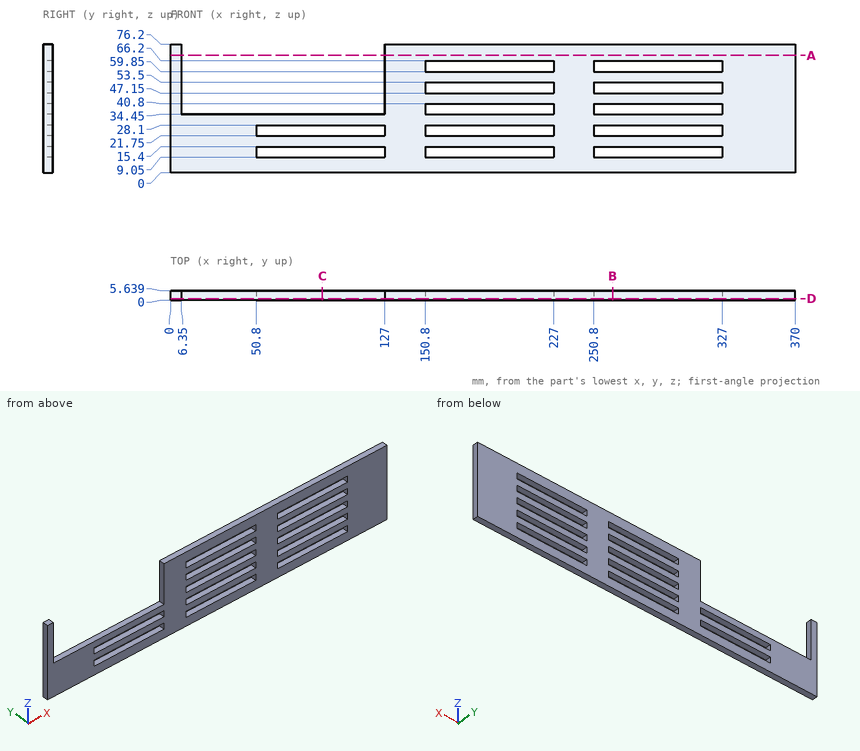
Part print with two shaded views. Sizes in mm from the minimum x, y, z corner. Round coordinates to 2 decimals unless told otherwise and drop trailing zeros. Order: outer loops, then holes, each group sorted by start corner. A loop starts at its lowest first (then second) coordinate and runs counter-clockwise, first axis right, second up. Notation, with made-up numbers: (71.25, 70) - (118.25, 70) arc R23 ccw to (118.25, 106) - close; hole circle Ø5 at (84.25, -26). An arc over 180 degrees is marked (long way). Answer in a Markdown table with one row per item. Add a question column.
(1) Probe L1, parallel to Z at x = 225, y = 0.7; L2, parallel to X at y = 4.7, z = 52.5; L3, parallel to Z at x = 115.5, y = 4.35. List the from-to ranges inside material, lowest first. Write a range as [from, to].
(2) Band-saw the part on C-C on x = 90. List the corners of the cut face in (y, z), and give its area (3 significant figures).
(3) Band-saw the part on A-A on z = 69.5. List the corners of the cut face in (x, y), and give its area (3 significant figures).
(4) Band-saw the part on B-B on x = 262. List the corners of the cut face in (y, z).
(5) Band-saw the part on D-D on y = 0.9. Count the separate pieces of the cut face and the enclosed holes in it, and give its area (4 significant figures).
Data:
| question | item | result |
|---|---|---|
| 1 | L1 | z = [0, 9.05], [15.4, 21.75], [28.1, 34.45], [40.8, 47.15], [53.5, 59.85], [66.2, 76.2] |
| 1 | L2 | x = [0, 6.35], [127, 150.8], [227, 250.8], [327, 370] |
| 1 | L3 | z = [0, 9.05], [15.4, 21.75], [28.1, 34.45] |
| 2 | outline | (0, 0) - (5.64, 0) - (5.64, 9.05) - (0, 9.05) - close; (0, 15.4) - (5.64, 15.4) - (5.64, 21.75) - (0, 21.75) - close; (0, 28.1) - (5.64, 28.1) - (5.64, 34.45) - (0, 34.45) - close |
| 2 | area | 123 mm^2 |
| 3 | outline | (0, 0) - (6.35, 0) - (6.35, 5.64) - (0, 5.64) - close; (127, 0) - (370, 0) - (370, 5.64) - (127, 5.64) - close |
| 3 | area | 1,410 mm^2 |
| 4 | outline | (0, 0) - (5.64, 0) - (5.64, 9.05) - (0, 9.05) - close; (0, 15.4) - (5.64, 15.4) - (5.64, 21.75) - (0, 21.75) - close; (0, 28.1) - (5.64, 28.1) - (5.64, 34.45) - (0, 34.45) - close; (0, 40.8) - (5.64, 40.8) - (5.64, 47.15) - (0, 47.15) - close; (0, 53.5) - (5.64, 53.5) - (5.64, 59.85) - (0, 59.85) - close; (0, 66.2) - (5.64, 66.2) - (5.64, 76.2) - (0, 76.2) - close |
| 5 | separate pieces | 1 |
| 5 | enclosed holes | 12 |
| 5 | area | 17,350 mm^2 |
